CAD build for the part. Positions are in the model's coordinates, mm. Face numbers are marked on the shaded views. A direction names the side the tool comes from. Give positions to 0.01 mm unless a question says otherwise; leave off trailing zeros. Write each loop counter-clockwise with the first axis right and the second up, starting at its lowest first coordinate (ties: lowest second). Pieces come first, ordered by that corner, then holes. Notation, with made-up numbers: (16.25, -29) - (29.25, -29) arc R20 ccw to (29.25, 2) - close; hole circle Ø10 at (73.5, 87). An arc over 180 degrees is marked (long way). Put each result on its own line as item: value. Start each with the question number.
1. Tool access for the marked faces 4, 5 and 6: list every direction of +Z, -Z, +X, -X, +Y, -Y with a clear straight run to the whole face (end or side of a thin tool).
2. Drop flat-ended pins along their axis: pin 1 (1.5 mm diameter, centred on x = 28, y = -3.5, fed in from +Z); pin 2 (6 mm diameter, centred on x = 16.5, y = -2.5, fed in from -Z); pin 3 (8.5 mm diameter, centred on x = -2.5, y = -2.5, fed in from +Z). Give the stop position or say it passes through.
3. Cut at C-C on y = -15. List the corners of the cut face in (x, z).
4. Cut at D-D on x = 24.5. List the corners of the cut face in (y, z).
5. Mould opens along Y. For the marked faces 1, 2 and 3 say: +Y half, -Y half, draft (parallel to the pull), parting line (faces both ways), or undercut.
6. Cut at A-A on z = 11. List the corners of the cut face in (x, y).
7. Wall check: line 1 (Y direction, x = 3, z = 13); line 2 (X direction, y = -4.5, z = 27.5); line 3 (X direction, y = 0, z = 13). Give the ranges that are in metal, low to high.
8. Cut at B-B on x = -15. List the corners of the cut face in (y, z), and give its area (3 significant figures).
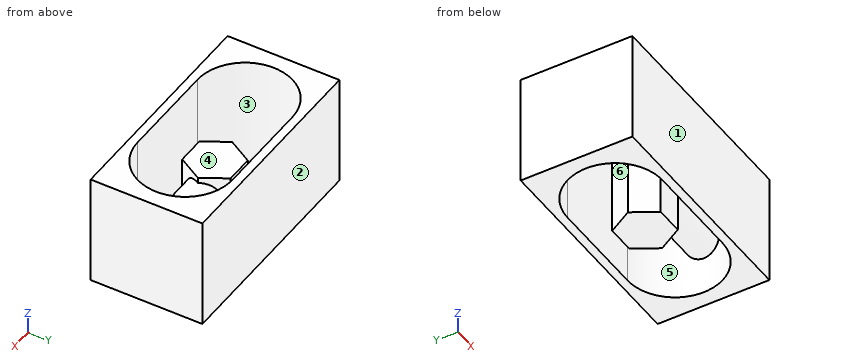
from build123d import *

# Parameters (mm, degrees)
SKETCH_W     = 80
SKETCH_H     = 40
PAD_DEPTH    = 40
POCKET_DEPTH = 40.001
SKETCH002_R  = 6.227756
PAD001_DEPTH = 40
PAD002_DEPTH = 28


with BuildPart() as part:
    # Sketch → Pad (new body)
    with BuildSketch(Plane.XY):
        Rectangle(SKETCH_W, SKETCH_H)
    extrude(amount=PAD_DEPTH)

    # Sketch001 (on Face6 of Pad) → Pocket (cut, through all)
    with BuildSketch(Plane.XY.offset(40)):
        with BuildLine():
            ThreePointArc((-17.5, 17), (-34.5, 0), (-17.5, -17))
            Line((-17.5, -17), (17.5, -17))
            ThreePointArc((17.5, -17), (34.5, 0), (17.5, 17))
            Line((-17.5, 17), (17.5, 17))
        make_face()
    extrude(amount=-POCKET_DEPTH, mode=Mode.SUBTRACT)

    # Sketch002 (on Face3 of Pocket) → Pad001 (join)
    with BuildSketch(Plane.YZ.offset(40)):
        with Locations((0, 19.750887)):
            Circle(SKETCH002_R)
    extrude(amount=-PAD001_DEPTH)

    # Sketch003 → Pad002 (join)
    with BuildSketch(Plane.XY):
        Polygon((10, 0), (5, 8.660254), (-5, 8.660254), (-10, 0), (-5, -8.660254), (5, -8.660254), align=None)
    extrude(amount=PAD002_DEPTH)


solid = part.part
Report:
1. face 4: +Z
1. face 5: none
1. face 6: +Z, -Z
2. pin 1: stops at z = 25.34
2. pin 2: stops at z = 13.52
2. pin 3: stops at z = 28
3. outline: (-40, 0) - (-25.5, 0) - (-25.5, 40) - (-40, 40) - close; (25.5, 0) - (40, 0) - (40, 40) - (25.5, 40) - close
4. outline: (-20, 0) - (-15.49, 0) - (-15.49, 40) - (-20, 40) - close; circle Ø12.46 at (0, 19.75); (15.49, 0) - (20, 0) - (20, 40) - (15.49, 40) - close
5. face 1: -Y half
5. face 2: +Y half
5. face 3: undercut
6. outline: (-40, -20) - (40, -20) - (40, 20) - (-40, 20) - close; (-10, 0) - (-5, -8.66) - (5, -8.66) - (10, 0) - (5, 8.66) - (-5, 8.66) - close; hole (-17.5, -17) - (17.5, -17) arc R17 ccw to (17.5, 17) - (-17.5, 17) arc R17 ccw to start
7. line 1: y = -20 to -17, -8.66 to 8.66, 17 to 20
7. line 2: x = -40 to -33.89, -7.4 to 7.4, 33.89 to 40
7. line 3: x = -40 to -34.5, -10 to 10, 34.5 to 40
8. outline: (-20, 0) - (-17, 0) - (-17, 40) - (-20, 40) - close; (17, 0) - (20, 0) - (20, 40) - (17, 40) - close
8. area: 240 mm²
